```python
from build123d import *

# Parameters (mm, degrees)
F0_W        = 64
F0_H        = 60
F1_DEPTH    = 35
F2_T        = -2
F3_R        = 5.08
F4_T1_DEPTH = 89.4
F5_R        = 2.54


# Not quite as in the source:
# - a fillet or chamfer that OpenCascade refuses, or shapes differently, is made with other operations: its cross-section is extruded or revolved along the edge and cut away or added


with BuildPart() as f1:
    # F0 (on Front) → F1 (new body)
    with BuildSketch(Plane.XZ):
        with Locations((-1.7414748222, 19.6752779907)):
            Rectangle(F0_W, F0_H)
    extrude(amount=F1_DEPTH)

    # F2
    f2_openings = [f1.faces().sort_by_distance(p)[0] for p in [
        (-1.741475, -17.5, -10.324722),
    ]]
    offset(amount=F2_T, openings=f2_openings)

    # F3
    f3_edges = [f1.edges().sort_by_distance(p)[0] for p in [
        (-1.741475, 0, 49.675278),
    ]]
    fillet(f3_edges, radius=F3_R)

    # F4: fillet of radius 5.08 on 1 edges, made by hand

    # F4_s2 → F4_t1 (cut)
    with BuildSketch(Plane.YZ.offset(-46.4414748222)):
        with BuildLine():
            ThreePointArc((0, -5.2447220093), (-1.4878975516, -8.8368244577), (-5.08, -10.3247220093))
            Line((-5.08, -10.3247220093), (0, -10.3247220093))
            Line((0, -10.3247220093), (0, -5.2447220093))
        make_face()
    extrude(amount=F4_T1_DEPTH, mode=Mode.SUBTRACT)

    # F5
    f5_edges = [f1.edges().sort_by_distance(p)[0] for p in [
        (-33.741475, -35, 19.675278),
        (30.258525, -35, 19.675278),
    ]]
    fillet(f5_edges, radius=F5_R)


solid = f1.part
```
Part model, mm, in its own coordinate system. A direction names the side the tool comes from. Round coordinates to 2 decimals unless told otherwise and drop trailing zeros. Loops run counter-clockwise (first coordinate to the right, second up) from the corner with the lowest first, then second, coordinate; pieces in that order, holes last. Notation, with made-up numbers: (76.5, -36.75) -> (103.5, -36.75) arc R27 ccw to (103.5, -11.75) -> close; hole circle Ø3 at (-2, 19). An arc over 180 degrees is marked (long way). Use CSV: the item, a comma, the result in double quotes. Start each with the question number.
1) Cut at D-D, the plane y = -3.5. Write the cut outline in (x, z), plus the area to 3 significant figures.
2) Drop a flat-ended pin along its axis: P1, Ø1.5, axis at x = -8, y = -14.5, coming from the -Z side. Give the stop position or say it passes through.
3) Cut at A-A, the plane z = 38.5. Write the cut outline in (x, y).
4) Which spindle directions (+Z, -Z, +X, -X, +Y, -Y) get a long thin tool onto all of the face, cutting with end or side? Do faces 5 (the flat face through (-2, -33, 19)), 6 (the flat face through (30.259, -16, 19)). Say none if no direction does.
5) Wall check: L1, parallel to X at y = -23, z = 3.5; L2, parallel to Y at x = -20.5, z = 15.5; L3, parallel to Z at x = 9, y = -14.5. Give the ranges that are in metal, low to high. Write a range as [from, to].
6) Cut at C-C, the plane x = 13. Write the cut outline in (y, z).
7) Pull direction X, two halves, no side cores. Call faces 1 (the cylindrical face through (29.49, -34.28, 20.1)), 2 (the flat face through (-2, -35, 20)), 3 (the flat face through (-2, -17, 47.675)), 4 (the flat face through (-33.741, -16, 19)): +X half, -X half, draft (parallel to the pull), parting line (faces both ways), or undercut.
8) Cut at B-B, the plane y = -9. Write the cut outline in (x, z), plus the area to 3 significant figures.
Determined:
1,outline,"(-33.74, -10.07) -> (-31.74, -10.07) -> (-31.74, 47.68) -> (28.26, 47.68) -> (28.26, -10.07) -> (30.26, -10.07) -> (30.26, 49.42) -> (-33.74, 49.42) -> close"
1,area,"343 mm2"
2,P1,"stops at z = 47.68"
3,outline,"(-33.74, -32.46) arc R2.54 ccw to (-31.2, -35) -> (27.72, -35) arc R2.54 ccw to (30.26, -32.46) -> (30.26, 0) -> (-33.74, 0) -> close; hole (-31.74, -33) -> (28.26, -33) -> (28.26, -2) -> (-31.74, -2) -> close"
4,face 5,"-Z"
4,face 6,"+Z, -Z, +X, +Y, -Y"
5,L1,"x = [-33.74, -31.74], [28.26, 30.26]"
5,L2,"y = [-35, -33], [-2, 0]"
5,L3,"z = [47.68, 49.68]"
6,outline,"(-35, -10.32) -> (-33, -10.32) -> (-33, 47.68) -> (-2, 47.68) -> (-2, -9.28) arc R5.08 ccw to (0, -5.24) -> (0, 44.6) arc R5.08 ccw to (-5.08, 49.68) -> (-35, 49.68) -> close"
7,face 1,"+X half"
7,face 2,"draft"
7,face 3,"undercut"
7,face 4,"-X half"
8,outline,"(-33.74, -10.32) -> (-31.74, -10.32) -> (-31.74, 47.68) -> (28.26, 47.68) -> (28.26, -10.32) -> (30.26, -10.32) -> (30.26, 49.68) -> (-33.74, 49.68) -> close"
8,area,"360 mm2"
